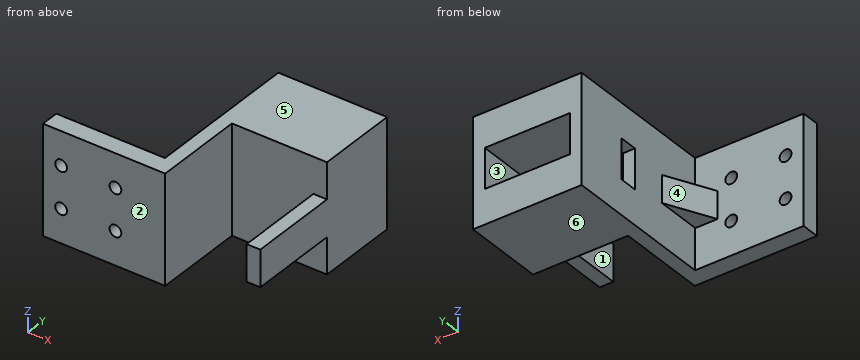
Autodesk Inventor part; units mm, degrees
ref_plane "YZ Plane" through (0, 0, 0) normal (1, 0, 0) x (0, 1, 0)
ref_plane "XZ Plane" through (0, 0, 0) normal (0, 1, 0) x (-1, 0, 0)
ref_plane "XY Plane" through (0, 0, 0) normal (0, 0, 1) x (1, 0, 0)
sketch "Boceto2" plane through (0, 0, 0) normal (0, 1, 0) x (-1, 0, 0)
  line L0 (-30, 30) -> (30, 30)
  line L1 (30, 30) -> (30, -30)
  line L2 (30, -30) -> (-30, -30)
  line L3 (-30, -30) -> (-30, 30)
  line L4 (-30, 30) -> (30, -30) construction
  line L5 (30, 30) -> (-30, -30) construction
  point P0 (0, 0)
  dimension "d0" = 60
  dimension "d1" = 60
extrude "Extrusión1" add sketch "Boceto2" along normal blind 55
sketch "Boceto3" plane through (30, 0, -30) normal (0, 0, -1) x (-1, 0, 0)
  line L0 (7.5, 50) -> (52.5, 50)
  line L1 (52.5, 50) -> (52.5, 0)
  line L2 (52.5, 0) -> (7.5, 0)
  line L3 (7.5, 0) -> (7.5, 50)
  line L4 (0, 0) -> (60, 0)
  point P0 (30, 0)
  dimension "d4" = 45
  dimension "d5" = 50
  dimension "d6" = 0
extrude "Extrusión2" cut sketch "Boceto3" against normal blind 190
sketch "Boceto5" plane through (0, 0, 0) normal (0, 1, 0) x (-1, 0, 0)
  line L0 (30, -30) -> (30, 30)
  line L1 (30, 0) -> (60, 0)
  line L2 (90, 30) -> (30, 30)
  line L3 (30, 30) -> (30, -30)
  line L4 (30, -30) -> (90, -30)
  line L5 (90, -30) -> (90, 30)
  line L6 (90, 30) -> (30, -30) construction
  line L7 (30, 30) -> (90, -30) construction
  circle A0 centre (50, 11.5) radius 3.25
  circle A1 centre (50, -11.5) radius 3.25
  circle A2 centre (80, 11.5) radius 3.25
  circle A3 centre (80, -11.5) radius 3.25
  point P0 (0, 0)
  dimension "d16" = 30
  dimension "d17" = 60
  dimension "d18" = 60
  dimension "d19" = 6.5
  dimension "d20" = 20
  dimension "d21" = 18.5
  dimension "d22" = 23
  dimension "d23" = 6.5
  dimension "d24" = 30
  dimension "d25" = 18.5
extrude "Extrusión4" add sketch "Boceto5" along normal blind 10
sketch "Boceto6" plane through (0, 55, 0) normal (0, 1, 0) x (1, 0, 0)
  line L0 (-30, 30) -> (-30, -30)
  line L1 (30, -30) -> (-30, -30)
  line L2 (-30, -30) -> (-30, 30)
  line L3 (-30, 30) -> (30, 30)
  line L4 (30, 30) -> (30, -30)
  line L5 (30, -30) -> (-30, 30) construction
  line L6 (-30, -30) -> (30, 30) construction
  point P0 (0, 0)
  dimension "d28" = 60
extrude "Extrusión5" add sketch "Boceto6" along normal blind 40
sketch "Boceto7" plane through (0, 95, 0) normal (0, 1, 0) x (1, 0, 0)
  line L0 (-23.5, 11) -> (23.5, 11)
  line L1 (23.5, 11) -> (23.5, -11)
  line L2 (23.5, -11) -> (-23.5, -11)
  line L3 (-23.5, -11) -> (-23.5, 11)
  line L4 (-23.5, 11) -> (23.5, -11) construction
  line L5 (23.5, 11) -> (-23.5, -11) construction
  point P0 (0, 0)
  dimension "d31" = 47
  dimension "d32" = 22
extrude "Extrusión6" cut sketch "Boceto7" against normal blind 43
sketch "Boceto8" plane through (-30, 0, 30) normal (-1, 0, 0) x (0, 0, 1)
  line L0 (-60, 55) -> (-44, 55)
  line L1 (0, 55) -> (-16, 55)
  line L2 (-44, 55) -> (-16, 55)
  line L3 (-41, 65) -> (-19, 65)
  line L4 (-19, 65) -> (-19, 55)
  line L5 (-19, 55) -> (-41, 55)
  line L6 (-41, 55) -> (-41, 65)
  line L7 (-41, 65) -> (-19, 55) construction
  line L8 (-19, 65) -> (-41, 55) construction
  line L9 (-16, 55) -> (-16, 95)
  line L10 (-44, 55) -> (-44, 95)
  point P0 (-30, 0)
  point P1 (-30, 60)
  point P2 (-41, 55)
  point P3 (-19, 55)
  point P4 (0, 95)
  point P5 (-60, 95)
  point P6 (-41, 60)
  dimension "d35" = 22
  dimension "d36" = 10
  dimension "d37" = 0
  dimension "d53" = 3
  dimension "d54" = 3
extrude "Extrusión7" cut sketch "Boceto8" against normal blind 10
ref_plane "Plano de trabajo1" through (30, 55, 0) normal (0, 0, -1) x (-1, 0, 0)
sketch "Boceto10" plane through (30, 55, 0) normal (0, 0, -1) x (-1, 0, 0)
  line L0 (60.12, -45) -> (60.12, 17.4198)
  line L1 (60.12, -45) -> (60.12, 13.5667)
  line L2 (60.12, -45) -> (137.1989, -45)
  line L3 (60.12, -19.9519) -> (80.5233, -61.6073)
  line L4 (120, -45) -> (60, -45)
  point P0 (30, -55)
  point P1 (72.3889, -45)
  dimension "d41" = 0
extrude "Extrusión8" add sketch "Boceto10" along normal mid plane 15
sketch "Boceto11" plane through (30, 0, 30) normal (1, 0, 0) x (0, 0, -1)
  line L0 (30, 0) -> (30, 50)
  line L1 (60, 50) -> (0, 50)
  line L2 (0, 0) -> (60, 0)
  line L3 (20, 50) -> (40, 50)
  line L4 (40, 50) -> (40, 0)
  line L5 (40, 0) -> (20, 0)
  line L6 (20, 0) -> (20, 50)
  line L7 (20, 50) -> (40, 0) construction
  line L8 (40, 50) -> (20, 0) construction
  line L9 (60, 0) -> (60, 95)
  line L10 (40, 50) -> (60, 50)
  line L11 (60, 50) -> (60, 0)
  line L12 (60, 0) -> (40, 0)
  line L13 (40, 0) -> (40, 50)
  line L14 (0, 0) -> (0, 95)
  line L15 (19.8706, 50) -> (0, 50)
  line L16 (0, 50) -> (0, 0)
  line L17 (0, 0) -> (19.8706, 0)
  line L18 (19.8706, 0) -> (19.8706, 50)
  point P0 (30, 25)
  dimension "d55" = 20
extrude "Extrusión9" cut sketch "Boceto11" against normal blind 10 contours L4 L1 L9 L2 | L2 L14 L1 L18
properties part number "depth_camera_support_v2"
CAD build for the part. Positions are in the model's coordinates, mm. Face numbers are marked on the shaded views. A direction names the side the tool comes from. Give positions to 0.01 mm unless a question says otherwise; leave off trailing zeros. Loops run counter-clockwise (first coordinate to the right, second up) from the corner with the lowest first, then second, coordinate; pieces in that order, holes last. Notation, with made-up numbers: (20.5, 76.5) -> (45.5, 76.5) arc R25 cw to (45.5, 104.5) -> close; hole circle Ø4 at (11.5, 71.5). An arc over 180 degrees is marked (long way). Use a Markdown table: item, result.
1. Mould opens along Z. For the marked faces 3, 4, 5 and 6 say: pulls with the +Z half, pulls with the -Z half, needs draft (parallel to the pull), parting line crosses it, or undercut.
Check result:
| item | result |
|---|---|
| face 3 | undercut |
| face 4 | needs draft |
| face 5 | pulls with the +Z half |
| face 6 | pulls with the -Z half |
2. Which spindle directions (+Z, -Z, +X, -X, +Y, -Y) get a long thin tool onto all of the face, cutting with end or side? Do the marked faces 1 and 2. Say none if no direction does.
Check result:
| item | result |
|---|---|
| face 1 | +Z, -Z, -Y |
| face 2 | +Z, -Z, +X, -X, -Y |
3. Slice it at A-A (z = 2). List the corners of the cut face in (x, y).
Check result:
| item | result |
|---|---|
| outline | (-90, 0) -> (-22.5, 0) -> (-22.5, 50) -> (22.5, 50) -> (22.5, 0) -> (30, 0) -> (30, 95) -> (23.5, 95) -> (23.5, 52) -> (-23.5, 52) -> (-23.5, 55) -> (-30, 55) -> (-30, 10) -> (-30.12, 10) -> (-30.12, 35.05) -> (-42.39, 10) -> (-90, 10) -> close; (-30, 65) -> (-23.5, 65) -> (-23.5, 95) -> (-30, 95) -> close |
4. Slice it at C-C (y = 44.5). List the corners of the cut face in (x, z), plus the area to 3 significant figures.
Check result:
| item | result |
|---|---|
| outline | (-30, -30) -> (-22.5, -30) -> (-22.5, 30) -> (-30, 30) -> close; (22.5, -10) -> (30, -10) -> (30, 10.13) -> (22.5, 10.13) -> close |
| area | 601 mm^2 |
5. Flat gauge pins, fed straight in: pin 1 (10.5 mm diameter, centred on x = -80, z = -11.5, fed in from +Y); pin 2 (3.5 mm diameter, centred on x = -37, y = 17.5, fed in from -Z); pin 3 (5 mm diameter, centred on y = 14.5, z = 21, fed in from -X). Where does each tip first touch, or does it go through?
Check result:
| item | result |
|---|---|
| pin 1 | stops at y = 10 |
| pin 2 | stops at z = -7.5 |
| pin 3 | stops at x = -30 |
6. Wall check: L1, parallel to Z at x = -80, y = 4; L2, parallel to X at y = 77, z = 0.5; L3, parallel to Y at x = -28.5, z = 5. Give the ranges that are in metal, low to high. Write a range as [from, to].
Check result:
| item | result |
|---|---|
| L1 | z = [-30, -14.75], [-8.25, 8.25], [14.75, 30] |
| L2 | x = [-30, -23.5], [23.5, 30] |
| L3 | y = [0, 55], [65, 95] |
7. Slice it at D-D (y = 80.5). List the corners of the cut face in (x, z), plus the area to 3 significant figures.
Check result:
| item | result |
|---|---|
| outline | (-30, -30) -> (30, -30) -> (30, 30) -> (-30, 30) -> close; hole (-23.5, -11) -> (23.5, -11) -> (23.5, 11) -> (-23.5, 11) -> close |
| area | 2,570 mm^2 |
8. Slice it at B-B (x = -50). List the corners of the cut face in (y, z), plus the area to 3 significant figures.
Check result:
| item | result |
|---|---|
| outline | (0, -30) -> (10, -30) -> (10, -14.75) -> (0, -14.75) -> close; (0, -8.25) -> (10, -8.25) -> (10, 8.25) -> (0, 8.25) -> close; (0, 14.75) -> (10, 14.75) -> (10, 30) -> (0, 30) -> close |
| area | 470 mm^2 |
